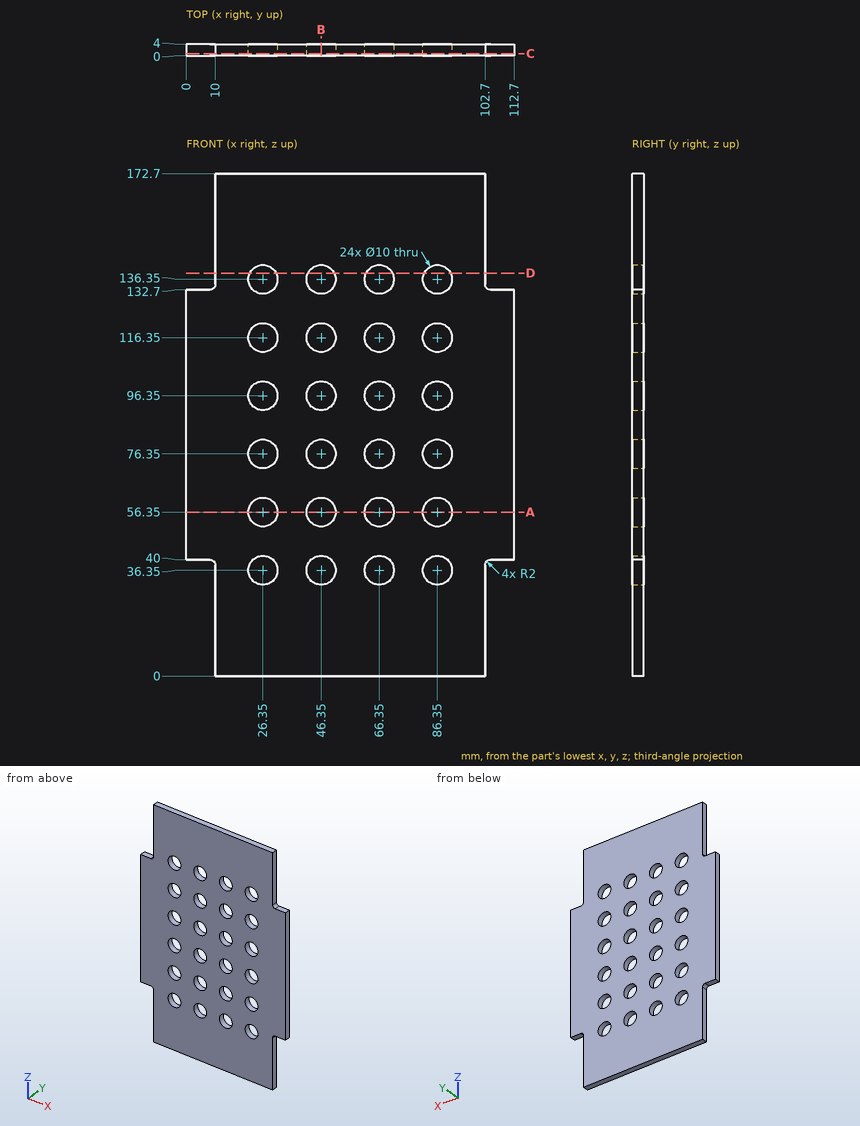
Study the drawing (mm; zero at the part's minimum x, y, z) and answer. Give positions to 0.01 mm unless a question says otherwise; leave off trailing zeros. Write each loop counter-clockwise with the first axis right and the second up, starting at its lowest first coordinate (ties: lowest second). Pieces come first, ordered by that corner, then holes. Notation, with made-up numbers: (69, -21.5) -> (111, -21.5) arc R9 ccw to (111, -7.5) -> close; hole circle Ø2 at (-22, 64.25). An arc over 180 degrees is marked (long way). Write item = value, one per line.
Q1. Section C-C on y = 0.7 is taken. State how many separate pieces and enclosed holes the cut face has, and give its area (3 significant figures).
Computed values:
separate_pieces = 1
enclosed_holes = 24
area = 16,000 mm^2
Q2. Section B-B on x = 46.35 is taken. Determine the outline of the cut face in (y, z), and give its area (3 significant figures).
Computed values:
outline = (0, 0) -> (4, 0) -> (4, 31.35) -> (0, 31.35) -> close; (0, 41.35) -> (4, 41.35) -> (4, 51.35) -> (0, 51.35) -> close; (0, 61.35) -> (4, 61.35) -> (4, 71.35) -> (0, 71.35) -> close; (0, 81.35) -> (4, 81.35) -> (4, 91.35) -> (0, 91.35) -> close; (0, 101.35) -> (4, 101.35) -> (4, 111.35) -> (0, 111.35) -> close; (0, 121.35) -> (4, 121.35) -> (4, 131.35) -> (0, 131.35) -> close; (0, 141.35) -> (4, 141.35) -> (4, 172.7) -> (0, 172.7) -> close
area = 451 mm^2
Q3. Consider line 1 along X through (y, z) = (2.95, 56.35); line 2 along X through (y, z) = (2, 36.35); line 3 along X through (y, z) = (0.8, 29.5). Determine where each line is inside the solid, lowest interval first.
Computed values:
line_1 = 0 to 21.35, 31.35 to 41.35, 51.35 to 61.35, 71.35 to 81.35, 91.35 to 112.7
line_2 = 10 to 21.35, 31.35 to 41.35, 51.35 to 61.35, 71.35 to 81.35, 91.35 to 102.7
line_3 = 10 to 102.7
Q4. Section D-D on z = 138.5 is taken. Determine the outline of the cut face in (x, y), and give its area (3 significant figures).
Computed values:
outline = (10, 0) -> (21.84, 0) -> (21.84, 4) -> (10, 4) -> close; (30.86, 0) -> (41.84, 0) -> (41.84, 4) -> (30.86, 4) -> close; (50.86, 0) -> (61.84, 0) -> (61.84, 4) -> (50.86, 4) -> close; (70.86, 0) -> (81.84, 0) -> (81.84, 4) -> (70.86, 4) -> close; (90.86, 0) -> (102.7, 0) -> (102.7, 4) -> (90.86, 4) -> close
area = 226 mm^2
Q5. Flat-ended cylindrical pins translate along their axes: pin 1 Ø1.2 at (x, y) = (2.5, 1) entering from -Z; pin 2 Ø2 at (x, y) = (107, 1.5) entering from +Z. Find the tip coordinate at first contact, or state that the pin passes through.
Computed values:
pin_1 = 40
pin_2 = 132.7
Q6. Section A-A on z = 56.35 is taken. Determine the outline of the cut face in (x, y).
Computed values:
outline = (0, 0) -> (21.35, 0) -> (21.35, 4) -> (0, 4) -> close; (31.35, 0) -> (41.35, 0) -> (41.35, 4) -> (31.35, 4) -> close; (51.35, 0) -> (61.35, 0) -> (61.35, 4) -> (51.35, 4) -> close; (71.35, 0) -> (81.35, 0) -> (81.35, 4) -> (71.35, 4) -> close; (91.35, 0) -> (112.7, 0) -> (112.7, 4) -> (91.35, 4) -> close
